```python
from build123d import *

# Parameters (mm, degrees)
SKETCH1_W           = 3
SKETCH1_H           = 1.5
SKETCH2_R           = 3.5
SKETCH2_R_2         = 1.495
BOSS_EXTRUDE1_DEPTH = 7.65
FILLET1_R           = 5
CHAMFER1_SIZE       = 1.9
BOSS_EXTRUDE2_DEPTH = 7.65
FILLET2_R           = 5


with BuildPart() as part:
    # Sketch1 → Revolve1 (revolve)
    with BuildSketch(Plane.XY):
        Polygon((-6.31640625, 27.5), (-6.31640625, 28.5), (1.33359375, 28.5), (1.33359375, 10.5), (0.33359375, 10.5), (0.33359375, 11.5), (-0.66640625, 11.5), (-0.66640625, 26.5), (-6.81640625, 26.5), (-6.81640625, 27.5), align=None)
        with Locations((-2.16640625, 12.25)):
            Rectangle(SKETCH1_W, SKETCH1_H)
    revolve(axis=Axis((0, 0, 0), (1, 0, 0)))

    # Sketch2 → Boss-Extrude1 (add)
    with BuildSketch(Plane.ZY.offset(6.31640625)):
        with Locations((-12.833666233, 27.116360579)):
            Circle(SKETCH2_R)
        with Locations((-12.833666233, 27.116360579)):
            Circle(SKETCH2_R_2, mode=Mode.SUBTRACT)
        with Locations((24.042513933, 17.943174852)):
            Circle(SKETCH2_R)
        with Locations((24.042513933, 17.943174852)):
            Circle(SKETCH2_R_2, mode=Mode.SUBTRACT)
        with Locations((15.464980443, -25.706699125)):
            Circle(SKETCH2_R)
        with Locations((15.464980443, -25.706699125)):
            Circle(SKETCH2_R_2, mode=Mode.SUBTRACT)
        with Locations((-25.706699125, -15.464980443)):
            Circle(SKETCH2_R)
        with Locations((-25.706699125, -15.464980443)):
            Circle(SKETCH2_R_2, mode=Mode.SUBTRACT)
    extrude(amount=-BOSS_EXTRUDE1_DEPTH)

    # Fillet1
    fillet1_edges = [part.edges().sort_by_distance(p)[0] for p in [
        (-2.49140625, 26.926500874, -9.338819556),
        (-2.49140625, 19.412851347, 20.866029871),
        (-2.49140625, -17.243063028, -22.691998092),
        (-2.49140625, -11.968566697, -25.865100255),
        (-2.49140625, -22.691998092, 17.243063028),
        (-2.49140625, -25.865100255, 11.968566697),
    ]]
    fillet(fillet1_edges, radius=FILLET1_R)

    # Chamfer1
    chamfer1_edges = [part.edges().sort_by_distance(p)[0] for p in [
        (1.33359375, 27.116360579, -14.328666233),
        (1.33359375, 17.943174852, 22.547513933),
        (1.33359375, -15.464980443, -27.201699125),
        (1.33359375, -25.706699125, 13.969980443),
    ]]
    chamfer(chamfer1_edges, length=CHAMFER1_SIZE)

    # Sketch4 → Boss-Extrude2 (add)
    with BuildSketch(Plane.ZY.offset(6.31640625)):
        with BuildLine():
            ThreePointArc((-14.902549995, 24.29329133), (-16.124726175, 25.925174422), (-16.230156511, 27.961259264))
            Line((-16.230156511, 27.961259264), (-17.61181157, 22.407009913))
            ThreePointArc((-17.61181157, 22.407009913), (-16.284515387, 23.38941125), (-14.902549995, 24.29329133))
        make_face()
        with BuildLine():
            Line((26.057349153, 11.544026816), (27.439004212, 17.098276167))
            ThreePointArc((27.439004212, 17.098276167), (26.391913334, 15.34888835), (24.547607559, 14.479812262))
            ThreePointArc((24.547607559, 14.479812262), (25.345021602, 13.033797605), (26.057349153, 11.544026816))
        make_face()
    extrude(amount=-BOSS_EXTRUDE2_DEPTH)

    # Fillet2
    fillet2_edges = [part.edges().sort_by_distance(p)[0] for p in [
        (-2.49140625, 22.407009913, -17.61181157),
        (-2.49140625, 11.544026816, 26.057349153),
    ]]
    fillet(fillet2_edges, radius=FILLET2_R)


solid = part.part
```
The model under review builds one solid part; all positions refer to its coordinate system, in mm. A direction names the side the tool comes from. Round coordinates to 2 decimals unless told otherwise and drop trailing zeros. Loops run counter-clockwise (first coordinate to the right, second up) from the corner with the lowest first, then second, coordinate; pieces in that order, holes last.
Item 1: For faces 1 (the face through (-3.784, 14.246, 22.345)), 2 (the face through (1.334, 1, 12)), list the 3-axis set-ups (+Z, -Z, +X, -X, +Y, -Y) from which the entire face can be reached by the end or side of a thin tool; tool diameter is ignored.
Determined:
face 1: -X
face 2: +Z, -Z, +X, +Y, -Y
Item 2: Clearance check with flat-ended pins moving along their axes: pin 1 Ø3.5 at (y, z) = (-15.46, -25.71) entering from +X; pin 2 Ø1.5 at (y, z) = (-9, 4) entering from -X; pin 3 Ø3 at (y, z) = (-13, 17) entering from -X. State where each tip first meets the part, or that it passes through.
Determined:
pin 1: stops at x = -0.31
pin 2: stops at x = 0.33
pin 3: stops at x = -0.67
Item 3: Take a section at C-C (x = -5.25). Give the number of separate pieces and of enclosed holes in the cut face, then the cut area to 3 significant figures.
Determined:
separate pieces: 1
enclosed holes: 5
area: 461 mm2
Item 4: Take a section at A-A (z = 0). Write out the cut boundary in (x, y).
Determined:
outline: (-6.82, -27.5) - (-6.32, -27.5) - (-6.32, -28.5) - (1.33, -28.5) - (1.33, -10.5) - (0.33, -10.5) - (0.33, -11.5) - (-3.67, -11.5) - (-3.67, -13) - (-0.67, -13) - (-0.67, -26.5) - (-6.82, -26.5) - close; (-6.82, 26.5) - (-0.67, 26.5) - (-0.67, 13) - (-3.67, 13) - (-3.67, 11.5) - (0.33, 11.5) - (0.33, 10.5) - (1.33, 10.5) - (1.33, 28.5) - (-6.32, 28.5) - (-6.32, 27.5) - (-6.82, 27.5) - close
Item 5: Mouldability with a two-part tool opening along Z and no side actions: class faces 3 (the face through (-2.545, 30.522, -13.643)), 4 (the face through (-2.44, 7.59, -27.47)), 5 (the face through (-2.44, -5.72, 27.92)), 6 (the face through (-2.4, -27.7, -6.7)) as released by +Z, released by -Z, zero draft, split by the parting line, or undercut.
Determined:
face 3: split by the parting line
face 4: released by -Z
face 5: released by +Z
face 6: undercut
Item 6: For line 1 (Z direction, x = -0.8, y = 0); line 2 (Y direction, x = -1, z = -7); line 3 (Y direction, x = -4.5, z = 0), list the stretches that pass through material, from the lowest coordinate up.
Determined:
line 1: z = -28.5 to -26.5, -13 to -11.5, 11.5 to 13, 26.5 to 28.5
line 2: y = -27.63 to -25.56, -10.95 to -9.12, 9.12 to 10.95, 25.56 to 27.87
line 3: y = -28.5 to -26.5, 26.5 to 28.5
